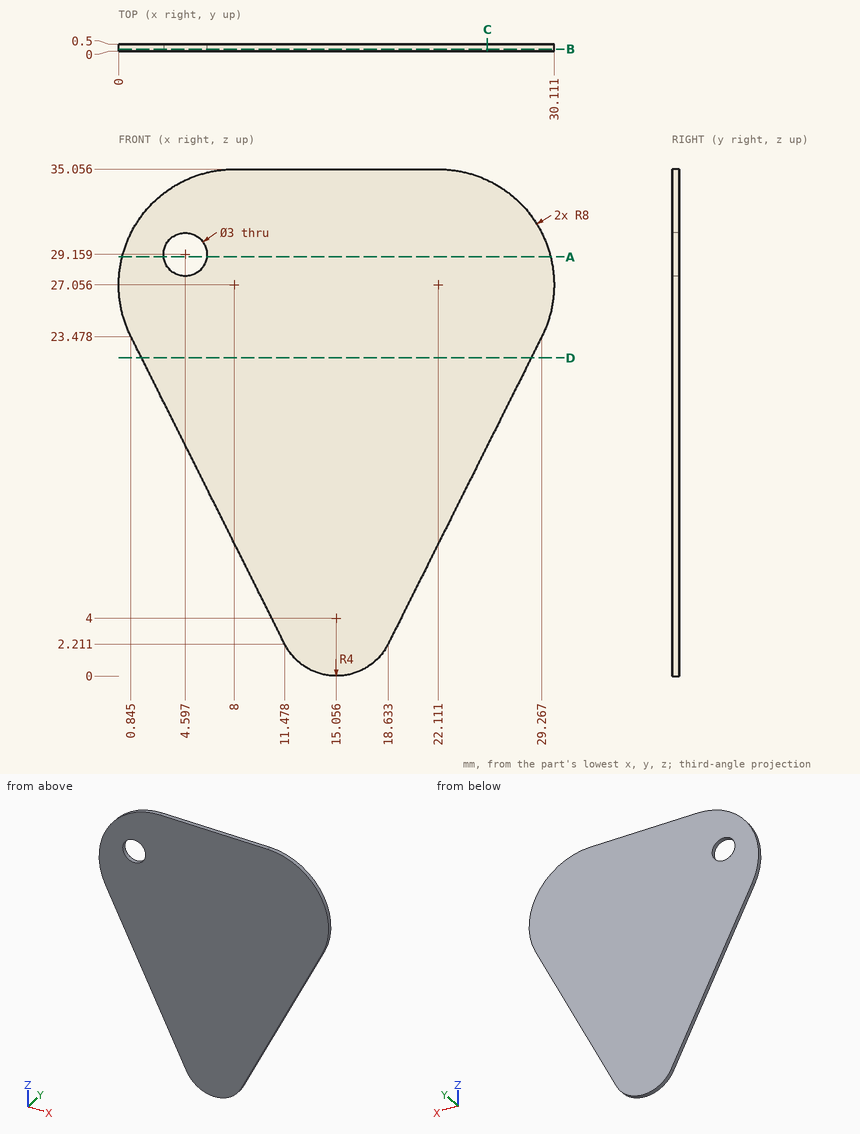
Geometry: see drawing. Coordinates: mm, zero at the bounding-box minimum. Round coordinates to 2 decimals unless told otherwise and drop trailing zeros. Loops run counter-clockwise (first coordinate to the right, second up) from the corner with the lowest first, then second, coordinate; pieces in that order, holes last. Notation, with made-up numbers: M 38.25,27 L 42.25,27 A31 cw 42.25,57 Z; hole C 11.5,9 d6. An arc over 180 degrees is marked long. Use a Markdown table: item, result. Add a question column.
1. Cut plane B-B, the plane y = 0.15. Output: boundary loops of the cut face in (x, z) (1 decimal).
2. Cut plane C-C, the plane x = 25.5. Output: boundary loops of the cut face in (y, z) (1 decimal).
3. Ray query, line 1 along Z through (x, y) = (3.5, 0.1) (1 decimal); line 2 along X through (y, z) = (0.4, 8) (1 decimal); line 3 along X through (y, z) = (0.2, 29) (1 decimal). Return the intervals inside material, ascending. Write a range as [from, to].
4. Cut plane A-A, the plane z = 29. Output: boundary loops of the cut face in (x, y) (1 decimal).
5. Cut plane D-D, the plane z = 22. Output: boundary loops of the cut face in (x, y).
Solution:
| question | item | result |
|---|---|---|
| 1 | outline | M 0.8,23.5 L 11.5,2.2 A4 ccw 18.6,2.2 L 29.3,23.5 A8 ccw 22.1,35.1 L 8,35.1 A8 ccw Z; hole C 4.6,29.2 d3 |
| 2 | outline | M 0,15.9 L 0.5,15.9 L 0.5,34.3 L 0,34.3 Z |
| 3 | line 1 | z = [18.2, 28.1], [30.2, 33.7] |
| 3 | line 2 | x = [8.6, 21.5] |
| 3 | line 3 | x = [0.2, 3.1], [6.1, 29.9] |
| 4 | outline | M 0.2,0 L 3.1,0 L 3.1,0.5 L 0.2,0.5 Z; M 6.1,0 L 29.9,0 L 29.9,0.5 L 6.1,0.5 Z |
| 5 | outline | M 1.58,0 L 28.53,0 L 28.53,0.5 L 1.58,0.5 Z |
